The model under review builds one solid part; all positions refer to its coordinate system, in mm. A direction names the side the tool comes from. Round coordinates to 2 decimals unless told otherwise and drop trailing zeros. Write each loop counter-clockwise with the first axis right and the second up, starting at its lowest first coordinate (ties: lowest second). Pieces come first, ordered by that corner, then holes. Notation, with made-up numbers: (-30, 16) - (8, 16) arc R24 cw to (8, 30) - close; hole circle Ø10 at (-23.5, 16.5). An arc over 180 degrees is marked (long way). Write each question's results on one line, items separated by ' | '.
```python
from build123d import *

# Parameters (mm, degrees)
SKETCH1_W                      = 44
SKETCH1_H                      = 44
SKETCH1_R                      = 2.05
SKETCH1_R_2                    = 10
BOSS_EXTRUDE1_DEPTH            = 5.5
SKETCH3_R                      = 11
CUT_EXTRUDE1_DEPTH             = 5.1
M4X0_7_TAPPED_HOLE1_AT_2_COUNT = 2
M4X0_7_TAPPED_HOLE1_AT_2_PITCH = 36
SKETCH6_R                      = 4.1
CUT_EXTRUDE2_DEPTH             = 7.5
SKETCH7_W                      = 44
SKETCH7_H                      = 44
SKETCH7_R                      = 12.5
SKETCH7_R_2                    = 4.1
CUT_EXTRUDE3_DEPTH             = 3
CUT_EXTRUDE_1_DEPTH            = 6
SKETCH_2_R                     = 2.05
CUT_EXTRUDE_2_DEPTH            = 5
CHAMFER_1_SIZE                 = 0.3


with BuildPart() as part:
    # Sketch1 → Boss-Extrude1 (new body, symmetric)
    with BuildSketch(Plane(origin=(0, 0, 0), x_dir=(1, 0, 0), z_dir=(0, 1, 0))):
        Rectangle(SKETCH1_W, SKETCH1_H)
        with Locations((0, 17)):
            Circle(SKETCH1_R, mode=Mode.SUBTRACT)
        with Locations((14.722431864, -8.5)):
            Circle(SKETCH1_R, mode=Mode.SUBTRACT)
        with Locations((-14.722431864, -8.5)):
            Circle(SKETCH1_R, mode=Mode.SUBTRACT)
        Circle(SKETCH1_R_2, mode=Mode.SUBTRACT)
    extrude(amount=BOSS_EXTRUDE1_DEPTH, both=True)

    # Sketch3 → Cut-Extrude1 (cut)
    with BuildSketch(Plane(origin=(0, 5.5, 0), x_dir=(1, 0, 0), z_dir=(0, 1, 0))):
        Circle(SKETCH3_R)
    extrude(amount=-CUT_EXTRUDE1_DEPTH, mode=Mode.SUBTRACT)

    # Sketch5 → M4x0.7 Tapped Hole1 (revolve, cut)
    with BuildSketch(Plane(origin=(-18, -1.5, -22), x_dir=(0, 1, 0), z_dir=(1, 0, 0))):
        Polygon((0, 0), (0, 7.991420021), (1.65, 7), (1.65, 0), align=None)
    m4x0_7_tapped_hole1 = revolve(axis=Axis((-18, -1.5, -28.35), (0, 0, 1)), mode=Mode.SUBTRACT)

    # M4x0.7 Tapped Hole1 at 2: M4x0.7 Tapped Hole1 ×2
    with Locations(*[(i * M4X0_7_TAPPED_HOLE1_AT_2_PITCH, 0, 0) for i in range(1, M4X0_7_TAPPED_HOLE1_AT_2_COUNT)]):
        add(m4x0_7_tapped_hole1, mode=Mode.SUBTRACT)

    # Mirror1: M4x0.7 Tapped Hole1 across plane
    add(m4x0_7_tapped_hole1.mirror(Plane.XY), mode=Mode.SUBTRACT)

    # Mirror1 copy 1 sketch → Mirror1 copy 1 (revolve, cut)
    with BuildSketch(Plane(origin=(18, -1.5, 22), x_dir=(0, 1, 0), z_dir=(1, 0, 0))):
        Polygon((0, 0), (0, -7.991420021), (1.65, -7), (1.65, 0), align=None)
    revolve(axis=Axis((18, -1.5, 28.35), (0, 0, 1)), mode=Mode.SUBTRACT)

    # Sketch6 → Cut-Extrude2 (cut)
    with BuildSketch(Plane(origin=(0, 5.5, 0), x_dir=(1, 0, 0), z_dir=(0, 1, 0))):
        with Locations((-14.722431864, -8.5)):
            Circle(SKETCH6_R)
        with Locations((0, 17)):
            Circle(SKETCH6_R)
        with Locations((14.722431864, -8.5)):
            Circle(SKETCH6_R)
    extrude(amount=-CUT_EXTRUDE2_DEPTH, mode=Mode.SUBTRACT)

    # Sketch7 → Cut-Extrude3 (cut)
    with BuildSketch(Plane(origin=(0, 5.5, 0), x_dir=(1, 0, 0), z_dir=(0, 1, 0))):
        Rectangle(SKETCH7_W, SKETCH7_H)
        Circle(SKETCH7_R, mode=Mode.SUBTRACT)
        with Locations((14.722431864, -8.5)):
            Circle(SKETCH7_R_2, mode=Mode.SUBTRACT)
        with Locations((0, 17)):
            Circle(SKETCH7_R_2, mode=Mode.SUBTRACT)
        with Locations((-14.722431864, -8.5)):
            Circle(SKETCH7_R_2, mode=Mode.SUBTRACT)
    extrude(amount=-CUT_EXTRUDE3_DEPTH, mode=Mode.SUBTRACT)

    # 草图1 → 切除-拉伸1 (cut)
    with BuildSketch(Plane.XZ.offset(5.5)):
        with BuildLine():
            Line((7, -36), (7, -16))
            ThreePointArc((7, -16), (10.5, -12.5), (14, -16))
            Line((14, -16), (14, -36))
            ThreePointArc((14, -36), (10.5, -39.5), (7, -36))
        make_face()
        with BuildLine():
            Line((-7, -36), (-7, -16))
            ThreePointArc((-7, -16), (-10.5, -12.5), (-14, -16))
            Line((-14, -16), (-14, -36))
            ThreePointArc((-14, -36), (-10.5, -39.5), (-7, -36))
        make_face()
        with BuildLine():
            Line((-7, 36), (-7, 16))
            ThreePointArc((-7, 16), (-10.5, 12.5), (-14, 16))
            Line((-14, 16), (-14, 36))
            ThreePointArc((-14, 36), (-10.5, 39.5), (-7, 36))
        make_face()
        with BuildLine():
            Line((7, 36), (7, 16))
            ThreePointArc((7, 16), (10.5, 12.5), (14, 16))
            Line((14, 16), (14, 36))
            ThreePointArc((14, 36), (10.5, 39.5), (7, 36))
        make_face()
    extrude(amount=-CUT_EXTRUDE_1_DEPTH, mode=Mode.SUBTRACT)

    # 草图2 → 切除-拉伸2 (cut)
    with BuildSketch(Plane.XZ.offset(-0.5)):
        with Locations((10.5, 18)):
            Circle(SKETCH_2_R)
        with Locations((-10.5, 18)):
            Circle(SKETCH_2_R)
        with Locations((-10.5, -18)):
            Circle(SKETCH_2_R)
        with Locations((10.5, -18)):
            Circle(SKETCH_2_R)
    extrude(amount=-CUT_EXTRUDE_2_DEPTH, mode=Mode.SUBTRACT)

    # 倒角1
    chamfer_1_edges = [part.edges().sort_by_distance(p)[0] for p in [
        (0, -5.5, 22),
        (18, -5.5, 22),
        (0, -5.5, -22),
        (-18, -5.5, -22),
        (14, -5.5, -19),
        (-7, -5.5, -19),
        (-14, -5.5, 19),
        (7, -5.5, 19),
        (10.5, -5.5, 12.5),
        (14, -5.5, 19),
        (14, -2.5, 22),
        (7, -2.5, 22),
        (-7, -5.5, 19),
        (-10, -5.5, 0),
        (-10.5, -5.5, 12.5),
        (-7, -2.5, 22),
        (-14, -2.5, 22),
        (-10.5, -5.5, -12.5),
        (-14, -5.5, -19),
        (-14, -2.5, -22),
        (-7, -2.5, -22),
        (7, -5.5, -19),
        (10.5, -5.5, -12.5),
        (7, -2.5, -22),
        (14, -2.5, -22),
        (-2.05, -5.5, -17),
        (8.45, 2.5, -18),
        (-12.55, 2.5, -18),
        (-12.55, 2.5, 18),
        (8.45, 2.5, 18),
        (12.672431864, -5.5, 8.5),
        (-16.772431864, -5.5, 8.5),
        (-11, 5.5, 0),
        (-18, -5.5, 22),
        (-22, -5.5, 0),
        (18, -5.5, -22),
        (22, -5.5, 0),
        (22, -1.5, 22),
        (-22, -1.5, 22),
        (-22, -1.5, -22),
        (22, -1.5, -22),
        (0, 2.5, 22),
        (-22, 2.5, 0),
        (0, 2.5, -22),
        (-4.1, 2.5, -17),
        (22, 2.5, 0),
        (10.622431864, 2.5, 8.5),
        (-12.5, 5.5, 0),
        (-18.822431864, 2.5, 8.5),
    ]]
    chamfer(chamfer_1_edges, length=CHAMFER_1_SIZE)


solid = part.part
```
Q1. The part is to be moulded in two halves that separate along X. For faces 6 (the flat face through (-14, -2, -19)), 7 (the flat face through (-10, -5.5, -5)), 8 (the flat face through (-22, -1, 0)), 9 (the flat face through (22, -1, 0)), say which applies: released by +X, released by -X, zero draft, split by the parting line, or undercut.
Evaluation:
face 6: undercut | face 7: zero draft | face 8: released by -X | face 9: released by +X
Q2. We need section D-D (y = 4). State the section outline as (x, z) points, plus the area to 3 significant figures.
Evaluation:
outline: circle Ø25 at (0, 0); hole circle Ø22 at (0, 0) | area: 111 mm^2
Q3. For probe 1 along X at (y, z) = (-4.05, -17); probe 2 along Z at (x, y) = (0, -1.45); probe 3 along Z at (x, y) = (0.5, 3.75), list the stretches that pass through material, from the lowest coordinate up.
Evaluation:
probe 1: x = -22 to -14, -7 to -2.05, 2.05 to 7, 14 to 22 | probe 2: z = -22 to -21.1, -12.9 to -10, 10 to 22 | probe 3: z = -12.49 to -10.99, 10.99 to 12.49
Q4. We need section A-A (z = 0). State the section outline as (x, y) points, plus the area to 3 significant figures.
Evaluation:
outline: (-22, -5.2) - (-21.7, -5.5) - (-10.3, -5.5) - (-10, -5.2) - (-10, 0.4) - (-11, 0.4) - (-11, 5.2) - (-11.3, 5.5) - (-12.2, 5.5) - (-12.5, 5.2) - (-12.5, 2.5) - (-21.7, 2.5) - (-22, 2.2) - close; (10, -5.2) - (10.3, -5.5) - (21.7, -5.5) - (22, -5.2) - (22, 2.2) - (21.7, 2.5) - (12.5, 2.5) - (12.5, 5.2) - (12.2, 5.5) - (11.3, 5.5) - (11, 5.2) - (11, 0.4) - (10, 0.4) - close | area: 196 mm^2
Q5. Tool access review of faces 1 (the cylindrical face through (-2.17, -2.44, 9.76)), 2 (the flat face through (14, -2, -19)), 3 (the cylindrical face through (16.61, -0.61, 18.55)), 4 (the conical face through (-18.28, -1.54, -14.18)), 5 (the flat face through (7, -2, 19)): name each direction out of +Z, -Z, +X, -X, +Y, -Y from which nothing blocks a thin tool from reaching the whole face with its end or side.
Evaluation:
face 1: +Y, -Y | face 2: -Z, -Y | face 3: +Z | face 4: -Z | face 5: +Z, -Y
Q6. We need section B-B (y = 1.25). State how many separate pieces and enclosed holes the cut face has, plus the area to 3 significant figures.
Evaluation:
separate pieces: 1 | enclosed holes: 8 | area: 1,340 mm^2
Q7. Insertion check: P1, Ø2.5, axis at x = -10.5, z = -18, coming from the +Y side; P2, Ø2.5, axis at x = 11.5, z = 15.5, coming from the -Y side; P3, Ø6.5, axis at x = -14.72, z = 8.5, coming from the +Y side. Each pin has a flat end and moves straight along its axis. Give the tip position at first contact, or say it passes through.
Evaluation:
P1: passes through | P2: stops at y = 0.5 | P3: stops at y = -2
